from build123d import *

# Parameters (mm, degrees)
BOSS_EXTRUDE1_DEPTH = 24
SKETCH2_R           = 4
SKETCH2_R_2         = 1.5
CUT_EXTRUDE1_DEPTH  = 19
CUT_EXTRUDE2_START  = -2
SKETCH3_R           = 4
SKETCH3_R_2         = 1.5
CUT_EXTRUDE2_DEPTH  = 2
FILLET1_R           = 12
SKETCH4_R           = 1.5
SKETCH4_R_2         = 4
CUT_EXTRUDE4_DEPTH  = 2
FILLET2_R           = 4


with BuildPart() as part:
    # Sketch1 → Boss-Extrude1 (new body)
    with BuildSketch(Plane.XY):
        Polygon((-78.301300665, 50.426714514), (-78.301300665, -5.573285486), (-26.301300665, -5.573285486), (-26.301300665, 50.426714514), (-24.301300665, 50.426714514), (-24.301300665, -7.573285486), (-80.301300665, -7.573285486), (-80.301300665, 50.426714514), align=None)
    extrude(amount=BOSS_EXTRUDE1_DEPTH)

    # Sketch2 → Cut-Extrude1 (cut)
    with BuildSketch(Plane(origin=(-24.301300665, 0, 0), x_dir=(0, 0, -1), z_dir=(1, 0, 0))):
        with Locations((-12, 37.426714514)):
            Circle(SKETCH2_R)
        with Locations((-4, 37.426714514)):
            Circle(SKETCH2_R_2)
        with Locations((-12, 29.426714514)):
            Circle(SKETCH2_R_2)
        with Locations((-20, 37.426714514)):
            Circle(SKETCH2_R_2)
        with Locations((-12, 45.426714514)):
            Circle(SKETCH2_R_2)
    extrude(amount=-CUT_EXTRUDE1_DEPTH, mode=Mode.SUBTRACT)

    # Sketch3 → Cut-Extrude2 (cut)
    with BuildSketch(Plane.ZY.offset(80.301300665).offset(CUT_EXTRUDE2_START)):
        with Locations(Location((12, 37.426714514, 0), (0, 0, 180))):
            Circle(SKETCH3_R)
        with Locations(Location((20, 37.426714514, 0), (0, 0, 180))):
            Circle(SKETCH3_R_2)
        with Locations(Location((12, 29.426714514, 0), (0, 0, 180))):
            Circle(SKETCH3_R_2)
        with Locations(Location((4, 37.426714514, 0), (0, 0, 180))):
            Circle(SKETCH3_R_2)
        with Locations(Location((12, 45.426714514, 0), (0, 0, 180))):
            Circle(SKETCH3_R_2)
    extrude(amount=CUT_EXTRUDE2_DEPTH, mode=Mode.SUBTRACT)

    # Fillet1
    fillet1_edges = [part.edges().sort_by_distance(p)[0] for p in [
        (-25.301300665, 50.426714514, 0),
        (-79.301300665, 50.426714514, 0),
        (-79.301300665, 50.426714514, 24),
        (-25.301300665, 50.426714514, 24),
    ]]
    fillet(fillet1_edges, radius=FILLET1_R - 0.0001)  # a hair under: the kernel refuses the full size

    # Sketch4 → Cut-Extrude4 (cut)
    with BuildSketch(Plane.XZ.offset(7.573285486)):
        with Locations(Location((-44.301300665, 12, 0), (0, 0, 270))):
            Circle(SKETCH4_R)
        with Locations(Location((-52.301300665, 4, 0), (0, 0, 270))):
            Circle(SKETCH4_R)
        with Locations(Location((-60.301300665, 12, 0), (0, 0, 270))):
            Circle(SKETCH4_R)
        with Locations(Location((-52.301300665, 12, 0), (0, 0, 270))):
            Circle(SKETCH4_R_2)
        with Locations(Location((-52.301300665, 20, 0), (0, 0, 270))):
            Circle(SKETCH4_R)
    extrude(amount=-CUT_EXTRUDE4_DEPTH, mode=Mode.SUBTRACT)

    # Fillet2
    fillet2_edges = [part.edges().sort_by_distance(p)[0] for p in [
        (-78.301300665, -5.573285486, 12),
        (-26.301300665, -5.573285486, 12),
        (-24.301300665, -7.573285486, 12),
        (-80.301300665, -7.573285486, 12),
    ]]
    fillet(fillet2_edges, radius=FILLET2_R)


solid = part.part
Can you work these out from the model? Positions are in its coordinate system, mm. A direction names the side the tool comes from. Round coordinates to 2 decimals unless told otherwise and drop trailing zeros. Loops run counter-clockwise (first coordinate to the right, second up) from the corner with the lowest first, then second, coordinate; pieces in that order, holes last. Notation, with made-up numbers: (-33.75, 12.25) - (4.25, 12.25) arc R27 cw to (4.25, 30.25) - close; hole circle Ø10 at (11.5, -19.75). An arc over 180 degrees is marked (long way). Answer in a Markdown table with one row per item. Add a question column.
Q1. I want a section at B-B on z = 20. List the corners of the cut face in (x, y) for me.
Q2. I need wall thicknesses on L1, parallel to X at y = -6, z = 12; L2, parallel to X at y = 24.5, z = 7; L3, parallel to Y at x = -25.4, z = 12. Which ranges of each line are inside material? Lowest first, please.
Q3. I want a section at A-A on y = 13.5. List the corners of the cut face in (x, z) for me, and give its area (3 significant figures).
Q4. Which directions (+Z, -Z, +X, -X, +Y, -Y) give clear straight access to the entire face, cutting with the end or side of a thin tool? Please do faces 1 (the flat face through (-57, -5.573, 12)), 2 (the cylindrical face through (-25.287, 46.914, 12.195)).
Q5. For pin 1 Ø1.8 at (x, z) = (-52.3, 4) entering from +Y; pin 2 Ø3.5 at (y, z) = (37.43, 20) entering from +X; pin 3 Ø10 at (x, z) = (-69.5, 15.5) entering from +Y, each with a flat end and sliding along its axis, tell me the tip position at first contact or that it passes through.
Q6. We'd pull the mould along Z, two halves only. Please class faces 3 (the cylindrical face through (-79.287, 47.005, 3.609)), 4 (the cylindrical face through (-25.287, 46.818, 20.578)), 5 (the cylindrical face through (-79.287, 44.413, 13.106)): pulls with the +Z half, pulls with the -Z half, needs draft (parallel to the pull), parting line crosses it, or undercut.
A:
| question | item | result |
|---|---|---|
| 1 | outline | (-80.3, -3.57) arc R4 ccw to (-76.3, -7.57) - (-53.8, -7.57) - (-53.8, -5.57) - (-74.3, -5.57) arc R4 cw to (-78.3, -1.57) - (-78.3, 35.93) - (-80.3, 35.93) - close; (-80.3, 38.93) - (-78.3, 38.93) - (-78.3, 47.37) - (-80.3, 47.37) - close; (-50.8, -7.57) - (-28.3, -7.57) arc R4 ccw to (-24.3, -3.57) - (-24.3, 35.93) - (-26.3, 35.93) - (-26.3, -1.57) arc R4 cw to (-30.3, -5.57) - (-50.8, -5.57) - close; (-26.3, 38.93) - (-24.3, 38.93) - (-24.3, 47.37) - (-26.3, 47.37) - close |
| 2 | L1 | -79.48 to -61.8, -58.8 to -56.3, -48.3 to -45.8, -42.8 to -25.12 |
| 2 | L2 | -80.3 to -78.3, -26.3 to -24.3 |
| 2 | L3 | -6.33 to 27.93, 30.93 to 33.43, 41.43 to 43.93, 46.93 to 50.43 |
| 3 | outline | (-80.3, 0) - (-78.3, 0) - (-78.3, 24) - (-80.3, 24) - close; (-26.3, 0) - (-24.3, 0) - (-24.3, 24) - (-26.3, 24) - close |
| 3 | area | 96.0 mm^2 |
| 4 | face 1 | +Z, -Z, +Y |
| 4 | face 2 | +X, -X |
| 5 | pin 1 | through |
| 5 | pin 2 | x = -24.3 |
| 5 | pin 3 | y = -5.57 |
| 6 | face 3 | pulls with the -Z half |
| 6 | face 4 | pulls with the +Z half |
| 6 | face 5 | undercut |
